For this review, take the finished solid that the model builds, in its own axes (mm). A direction names the side the tool comes from. Coordinates: 2 decimals unless noted, no trailing zeros. Write each loop counter-clockwise with the first axis right and the second up, starting at its lowest first coordinate (ties: lowest second). Pieces come first, ordered by that corner, then holes.
```python
from build123d import *

# Parameters (mm, degrees)
SKETCH_1_R          = 27.5
EXTRUDE_1_DEPTH     = 5
SKETCH_2_R          = 24
EXTRUDE_2_DEPTH     = 25
SKETCH_4_W          = 65
SKETCH_4_H          = 55
EXTRUDE_3_DEPTH     = 5
SKETCH_5_R          = 21
CUT_EXTRUDE_1_DEPTH = 59
FILLET_1_R          = 10
SKETCH_6_R          = 1.75
CUT_EXTRUDE_2_DEPTH = 10
FILLET_2_R          = 2


with BuildPart() as part:
    # 草图1 → 凸台-拉伸1 (new body)
    with BuildSketch(Plane.XY):
        Circle(SKETCH_1_R)
    extrude(amount=EXTRUDE_1_DEPTH)

    # 草图2 → 凸台-拉伸2 (add)
    with BuildSketch(Plane.XY.offset(5)):
        Circle(SKETCH_2_R)
    extrude(amount=EXTRUDE_2_DEPTH)

    # 草图4 → 凸台-拉伸3 (add)
    with BuildSketch(Plane(origin=(0, 0, 0), x_dir=(-1, 0, 0), z_dir=(0, 0, -1))):
        Rectangle(SKETCH_4_W, SKETCH_4_H)
    extrude(amount=-EXTRUDE_3_DEPTH)

    # 草图5 → 切除-拉伸1 (cut)
    with BuildSketch(Plane.XY.offset(30)):
        Circle(SKETCH_5_R)
    extrude(amount=-CUT_EXTRUDE_1_DEPTH, mode=Mode.SUBTRACT)

    # 圆角1
    fillet_1_edges = [part.edges().sort_by_distance(p)[0] for p in [
        (32.5, 27.5, 2.5),
        (-32.5, -27.5, 2.5),
        (32.5, -27.5, 2.5),
        (-32.5, 27.5, 2.5),
    ]]
    fillet(fillet_1_edges, radius=FILLET_1_R)

    # 草图6 → 切除-拉伸2 (cut)
    with BuildSketch(Plane.XY.offset(5)):
        with Locations((-25.5, -17.5)):
            Circle(SKETCH_6_R)
        with Locations((-25.5, 17.5)):
            Circle(SKETCH_6_R)
        with Locations((25.5, 17.5)):
            Circle(SKETCH_6_R)
        with Locations((25.5, -17.5)):
            Circle(SKETCH_6_R)
    extrude(amount=-CUT_EXTRUDE_2_DEPTH, mode=Mode.SUBTRACT)

    # 圆角2
    fillet_2_edges = [part.edges().sort_by_distance(p)[0] for p in [
        (-24, 0, 5),
    ]]
    fillet(fillet_2_edges, radius=FILLET_2_R)


solid = part.part
```
1) Consider section A-A (x = 0). Give the boundary of the cut face in (y, z), then the cut area to 3 significant figures.
2) Consider section C-C (z = 2.75). Give the boundary of the cut face in (x, y), then the cut area to 3 significant figures.
3) Consider section B-B (y = 0). Give the boundary of the cut face in (x, z).
4) Tool access review of faces 1 (the face through (20.03, 6.31, 15.21)), 2 (the face through (-23.977, 1.055, 18.339)): name each direction out of +Z, -Z, +X, -X, +Y, -Y from which nothing blocks a thin tool from reaching the whole face with its end or side.
5) For L1, parallel to X at y = -0.5, z = 21; L2, parallel to Y at x = -25.5, z = 1.55; L3, parallel to Y at x = 0, z = 7, list the stretches that pass through material, from the lowest coordinate up.
6) The part is to be moulded in two halves that separate along Y. For faces 3 (the face through (24.21, 18.68, 2.54)), 4 (the face through (-29.49, -24.65, 2.54)), 5 (the face through (29.65, 24.49, 2.54)), say which applies: pulls with the +Y half, pulls with the -Y half, needs draft (parallel to the pull), parting line crosses it, or undercut.
7) Clearance check with flat-ended pins moving along their axes: P1, Ø5.5, axis at x = -25.5, y = 17.5, coming from the -Z side; P2, Ø2, axis at y = 5.5, z = 23, coming from the +X side; P3, Ø1.5, axis at y = -15, z = 17, coming from the -X side; P4, Ø1, axis at y = 7, z = 10, coming from the +X side. State where each tip first meets the part, or that it passes through.
8) Consider section D-D (z = 22). Give the boundary of the cut face in (x, y), then the cut area to 3 significant figures.
Results:
1. outline: (-27.5, 0) - (-21, 0) - (-21, 30) - (-24, 30) - (-24, 7) arc R2 cw to (-26, 5) - (-27.5, 5) - close; (21, 0) - (27.5, 0) - (27.5, 5) - (26, 5) arc R2 cw to (24, 7) - (24, 30) - (21, 30) - close
1. area: 217 mm2
2. outline: (-32.5, -17.5) arc R10 ccw to (-22.5, -27.5) - (22.5, -27.5) arc R10 ccw to (32.5, -17.5) - (32.5, 17.5) arc R10 ccw to (22.5, 27.5) - (-22.5, 27.5) arc R10 ccw to (-32.5, 17.5) - close; hole circle Ø3.5 at (-25.5, -17.5); hole circle Ø3.5 at (-25.5, 17.5); hole circle Ø42 at (0, 0); hole circle Ø3.5 at (25.5, -17.5); hole circle Ø3.5 at (25.5, 17.5)
2. area: 2,070 mm2
3. outline: (-32.5, 0) - (-21, 0) - (-21, 30) - (-24, 30) - (-24, 7) arc R2 cw to (-26, 5) - (-32.5, 5) - close; (21, 0) - (32.5, 0) - (32.5, 5) - (26, 5) arc R2 cw to (24, 7) - (24, 30) - (21, 30) - close
4. face 1: +Z, -Z
4. face 2: +Z
5. L1: x = -23.99 to -20.99, 20.99 to 23.99
5. L2: y = -27.04 to -19.25, -15.75 to 15.75, 19.25 to 27.04
5. L3: y = -24 to -21, 21 to 24
6. face 3: undercut
6. face 4: pulls with the -Y half
6. face 5: pulls with the +Y half
7. P1: stops at z = 0
7. P2: stops at x = 23.57
7. P3: stops at x = -19.31
7. P4: stops at x = 23.1
8. outline: circle Ø48 at (0, 0); hole circle Ø42 at (0, 0)
8. area: 424 mm2
